The figure shows three views and two pictorial views of one solid part (mm, origin at its lowest corner). Answer the questions. A direction names the side the tool comes from. Coordinates: 2 decimals unless noted, no trailing zeros. Loops run counter-clockwise (first coordinate to the right, second up) from the corner with the lowest first, then second, coordinate; pieces in that order, holes last. Notation, with made-up numbers: (-28, 87.5) -> (-9, 87.5) arc R15 ccw to (-9, 100.5) -> close; hole circle Ø3 at (-39.5, 85). An arc over 180 degrees is marked (long way). Answer as a JSON object with one key per item and string values. Group by question number.
1) Section D-D, the plane z = 2 is taken. Give the vertices of the cut face in (x, y).
2) Section C-C, the plane x = 8 is taken. Give the vertices of the cut face in (y, z), plus the area to 3 significant figures.
3) Consider probe 1 along Z at (x, y) = (8, 13.75); probe 2 along Y at (x, z) = (1.65, 6.5); probe 3 along X at (y, z) = (0.75, 4.25). Determine where each line is inside the solid, lowest interval first. Write a range as [from, to].
4) Determine the mould class of the marked faces 3, 4 and 5 for opening direction Z: released by +Z, released by -Z, zero draft, split by the parting line, or undercut.
5) A flat-ended cylindrical pin translates along its axis: P1, Ø1.7, axis at y = 11.24, z = 10.74, coming from the +X side. Find the tip coordinate at first contact, or state that the pin passes through.
6) Section A-A, the plane z = 6.5 is taken. Give the vertices of the cut face in (x, y), plus the area to 3 significant figures.
7) Section B-B, the plane y = 7 is taken. Give the vertices of the cut face in (x, z), plus the area to 3 significant figures.
8) Which of the six approach directions +Z, -Z, +X, -X, +Y, -Y give full straight-line access (tool end or side, diameter ignored) to the marked faces 1 and 2?
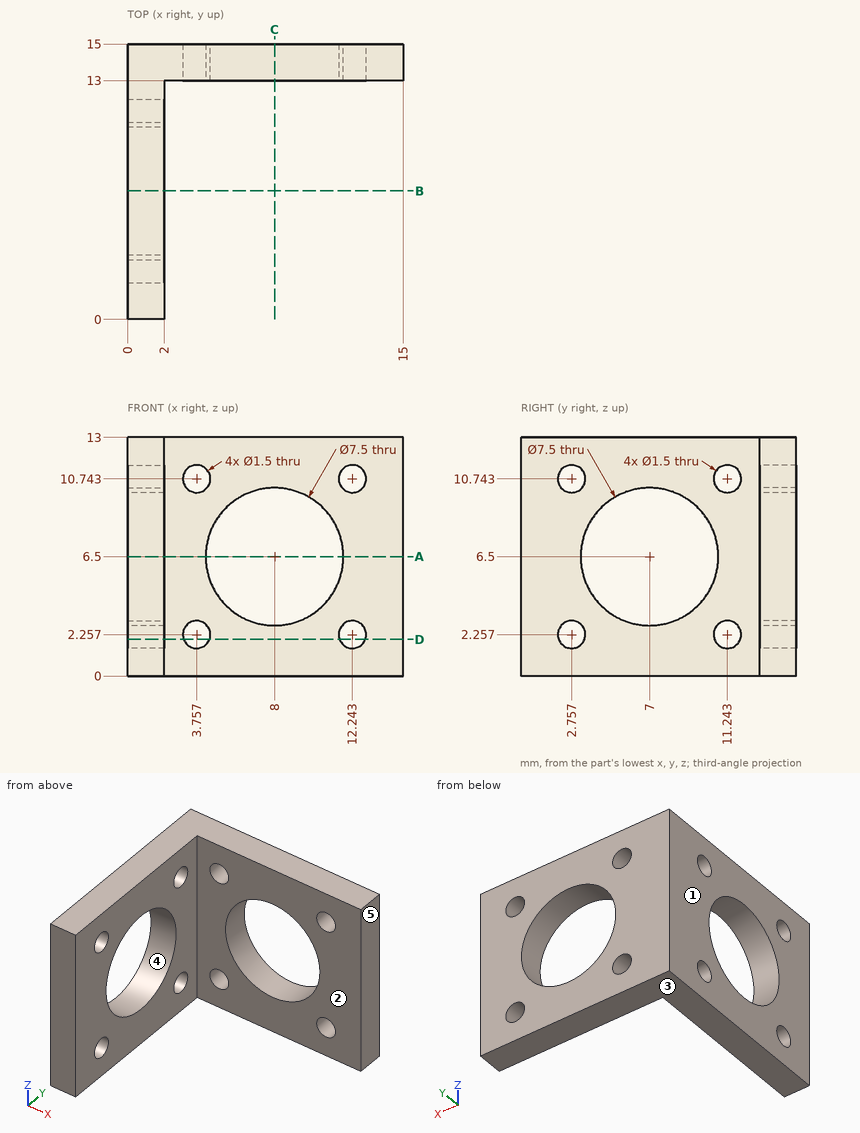
Determined:
{
 "1": {"outline": "(0, 0) -> (2, 0) -> (2, 2.05) -> (0, 2.05) -> close; (0, 3.46) -> (2, 3.46) -> (2, 10.54) -> (0, 10.54) -> close; (0, 11.95) -> (2, 11.95) -> (2, 13) -> (3.05, 13) -> (3.05, 15) -> (0, 15) -> close; (4.46, 13) -> (11.54, 13) -> (11.54, 15) -> (4.46, 15) -> close; (12.95, 13) -> (15, 13) -> (15, 15) -> (12.95, 15) -> close"},
 "2": {"outline": "(13, 0) -> (15, 0) -> (15, 2.75) -> (13, 2.75) -> close; (13, 10.25) -> (15, 10.25) -> (15, 13) -> (13, 13) -> close", "area": "11.0 mm²"},
 "3": {"probe 1": "[0, 2.75], [10.25, 13]", "probe 2": "[0, 3.25], [10.75, 15]", "probe 3": "[0, 2]"},
 "4": {"face 3": "released by -Z", "face 4": "undercut", "face 5": "zero draft"},
 "5": {"P1": "x = 2"},
 "6": {"outline": "(0, 0) -> (2, 0) -> (2, 3.25) -> (0, 3.25) -> close; (0, 10.75) -> (2, 10.75) -> (2, 13) -> (4.25, 13) -> (4.25, 15) -> (0, 15) -> close; (11.75, 13) -> (15, 13) -> (15, 15) -> (11.75, 15) -> close", "area": "26.0 mm²"},
 "7": {"outline": "(0, 0) -> (2, 0) -> (2, 2.75) -> (0, 2.75) -> close; (0, 10.25) -> (2, 10.25) -> (2, 13) -> (0, 13) -> close", "area": "11.0 mm²"},
 "8": {"face 1": "+Z, -Z, -X, +Y, -Y", "face 2": "+Z, -Z, +X, -Y"}
}
